```python
from build123d import *

# Parameters (mm, degrees)
CUT_EXTRUDE_1_DEPTH      = 31.298514815
CUT_EXTRUDE_1_DEPTH_BACK = 31.298514815
SKETCH_2_R               = 2.5
SKETCH_3_R               = 0.5
CUT_EXTRUDE_2_DEPTH      = 2
CHAMFER_1_SIZE           = 0.49


with BuildPart() as part:
    # Эскиз1 → Повернуть1 (revolve)
    with BuildSketch(Plane.XY):
        Polygon((0, -11.826368877), (0, 13.173631123), (-3, 13.173631123), (-3, -7.826368877), (-0.875, -7.826368877), (-0.875, -11.826368877), align=None)
        with BuildLine():
            Line((0, 13.173631123), (0, 18.173631123))
            Line((0, 18.173631123), (-0.875, 18.173631123))
            ThreePointArc((-0.875, 18.173631123), (-1.43264439, 15.459067489), (-3, 13.173631123))
            Line((-3, 13.173631123), (0, 13.173631123))
        make_face()
    revolve(axis=Axis((0, 18.173631123, 0), (0, -1, 0)))

    # Эскиз2 → Вырез-Вытянуть1 (cut, two sides: drawn at the far end of the back side and taken through both)
    with BuildSketch(Plane(origin=(0, 18.173631123, 0), x_dir=(1, 0, 0), z_dir=(0, 1, 0)).offset(-CUT_EXTRUDE_1_DEPTH_BACK)):
        with Locations((-3.464101615, 2)):
            Circle(SKETCH_2_R)
        with Locations((3.464101615, 2)):
            Circle(SKETCH_2_R)
        with Locations((0, -4)):
            Circle(SKETCH_2_R)
    extrude(amount=CUT_EXTRUDE_1_DEPTH + CUT_EXTRUDE_1_DEPTH_BACK, mode=Mode.SUBTRACT)

    # Эскиз3 → Вырез-Вытянуть2 (cut)
    with BuildSketch(Plane.XZ.offset(11.826368877)):
        Circle(SKETCH_3_R)
    extrude(amount=-CUT_EXTRUDE_2_DEPTH, mode=Mode.SUBTRACT)

    # Фаска1
    chamfer_1_edges = [part.edges().sort_by_distance(p)[0] for p in [
        (-0.5, -9.826368877, 0),
    ]]
    chamfer(chamfer_1_edges, length=CHAMFER_1_SIZE)


solid = part.part
```
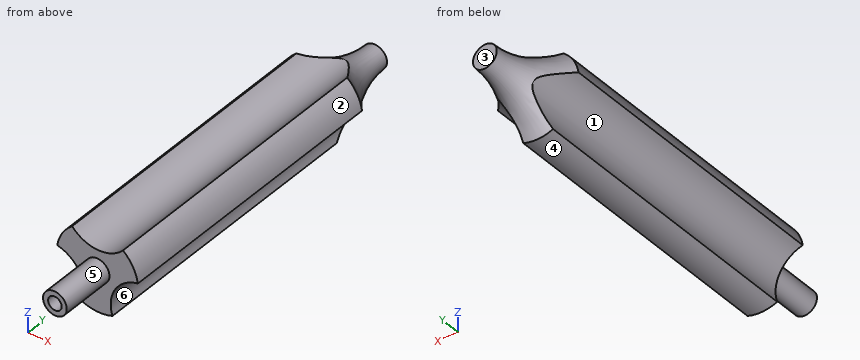
Geometry check sheet. Reference: the model listing, model coordinates, mm. Face numbers are marked on the shaded views. A direction names the side the tool comes from. Coordinates: 2 decimals unless noted, no trailing zeros. Order: outer loops, then holes, each group sorted by start corner. A loop starts at its lowest first (then second) coordinate and runs counter-clockwise, first axis right, second up.
Item 1: Mould release check, pull along Z, two halves, no side actions. Record for the marked faces 1, 2, 3 and 4: released by +Z, released by -Z, zero draft, split by the parting line, or undercut.
Item 2: Scan lines: line 1 along Z through (x, y) = (0, -11.1) (3 decimals); line 2 along X through (y, z) = (-2, 1.7); line 3 along Y through (x, z) = (-0.8, -2.3). Record each from-to range of solid material in increasing order.
Item 3: Section check B-B (y = 16.5). Enter the section's corners in (x, z).
Item 4: Tool access check on the marked faces 5 and 6. Record the directions out of +Z, -Z, +X, -X, +Y, -Y that give a thin tool (end or side, any length) a straight path to the whole face; none if there is none.
Item 5: Depth check by flat-ended pin: pin 1 (3 mm diameter, centred on y = 2, z = 0.5, fed in from +X); pin 2 (1 mm diameter, centred on y = 7, z = -1.5, fed in from +X). Enter the tip coordinate at first touch or a pass-through.
Item 6: Section check A-A (y = 3). Enter the section's corners in (x, z), plus the area to 3 significant figures.
Check sheet entries:
1. face 1: undercut
1. face 2: released by +Z
1. face 3: zero draft
1. face 4: released by -Z
2. line 1: z = -0.875 to -0.5, 0.5 to 0.875
2. line 2: x = -2.47 to -0.98, 0.98 to 2.47
2. line 3: y = -7.83 to 13.79
3. outline: circle Ø2.17 at (0, 0)
4. face 5: -Y
4. face 6: +X, +Y, -Y
5. pin 1: stops at x = 2.97
5. pin 2: stops at x = 1.17
6. outline: (-2.97, 0.45) arc R2.5 cw to (-1.09, -2.79) arc R3 ccw to (1.09, -2.79) arc R2.5 cw to (2.97, 0.45) arc R3 ccw to (1.87, 2.34) arc R2.5 cw to (-1.87, 2.34) arc R3 ccw to start
6. area: 16.7 mm2
